```python
from build123d import *

# Parameters (mm, degrees)
BATON_DEPTH       = 2.54
SKETCH5_R         = 1.905
JOINER_HOLE_DEPTH = 2.54


with BuildPart() as part:
    # Sketch1 → baton (new body)
    with BuildSketch(Plane(origin=(0, 0, 0), x_dir=(1, 0, 0), z_dir=(0, 1, 0))):
        with BuildLine():
            Line((-12.7, 5.08), (12.7, 5.08))
            ThreePointArc((12.7, 5.08), (17.78, 0), (12.7, -5.08))
            Line((12.7, -5.08), (-12.7, -5.08))
            ThreePointArc((-12.7, -5.08), (-17.78, 0), (-12.7, 5.08))
        make_face()
    extrude(amount=BATON_DEPTH)

    # Sketch5 → joiner hole (cut)
    with BuildSketch(Plane(origin=(0, 2.54, 0), x_dir=(1, 0, 0), z_dir=(0, 1, 0))):
        with Locations(Location((13.97, 0, 0), (0, 0, 270))):
            Circle(SKETCH5_R)
    extrude(amount=-JOINER_HOLE_DEPTH, mode=Mode.SUBTRACT)


solid = part.part
```
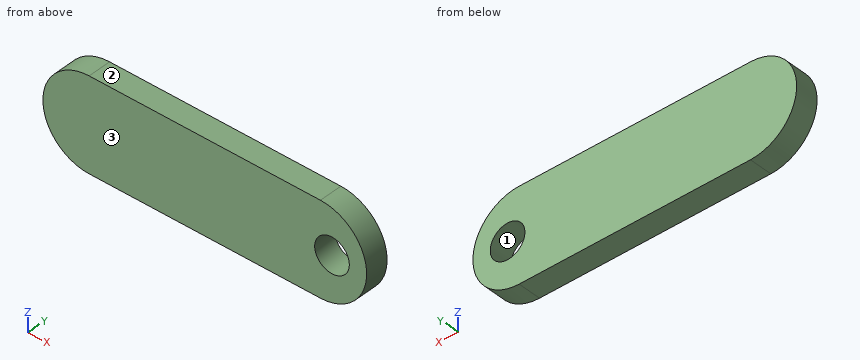
CAD build for the part. Positions are in the model's coordinates, mm. Face numbers are marked on the shaded views. Give positions to 0.01 mm unless a question says otherwise; leave off trailing zeros. Order: outer loops, then holes, each group sorted by start corner. A loop starts at its lowest first (then second) coordinate and runs counter-clockwise, first axis right, second up.
(1) Saw through at B-B, the plane y = 0.95. Give the cut face in (x, z) (3 decimals).
(2) Saw through at A-A, the plane z = 0. Give the cut face in (x, y) (3 decimals), then the cut area to 3 significant figures.
(3) Flat gauge pins, fed straight in: pin 1 (2.5 mm diameter, centred on x = 13.97, z = 0, fed in from -Y); pin 2 (1.5 mm diameter, centred on x = 2.5, z = 0, fed in from -Y). Where does each tip first touch, or does it go through?
(4) Saw through at D-D, the plane z = 2.5. Give the cut face in (x, y).
(5) Saw through at C-C, the plane x = 13.97. Give the cut face in (y, z) (3 decimals), then the cut area to 3 significant figures.
(6) Mould opens along Z. For the marked faces 1, 2 and 3 say: released by +Z, released by -Z, zero draft, split by the parting line, or undercut.
(7) Drill centre lines: L1, parallel to X at y = 1.95, z = 0 (3 decimals); L2, parallel to X at y = 1.35, z = 0.5; L3, parallel to X at y = 1, z = 4.5. Where is each one in solid material? Low to high.
Results found:
1. outline: (-12.7, -5.08) - (12.7, -5.08) arc R5.08 ccw to (12.7, 5.08) - (-12.7, 5.08) arc R5.08 ccw to start; hole circle Ø3.81 at (13.97, 0)
2. outline: (-17.78, 0) - (12.065, 0) - (12.065, 2.54) - (-17.78, 2.54) - close; (15.875, 0) - (17.78, 0) - (17.78, 2.54) - (15.875, 2.54) - close
2. area: 80.6 mm2
3. pin 1: passes through
3. pin 2: stops at y = 0
4. outline: (-17.12, 0) - (17.12, 0) - (17.12, 2.54) - (-17.12, 2.54) - close
5. outline: (0, -4.919) - (2.54, -4.919) - (2.54, -1.905) - (0, -1.905) - close; (0, 1.905) - (2.54, 1.905) - (2.54, 4.919) - (0, 4.919) - close
5. area: 15.3 mm2
6. face 1: undercut
6. face 2: released by +Z
6. face 3: zero draft
7. L1: x = -17.78 to 12.065, 15.875 to 17.78
7. L2: x = -17.76 to 12.13, 15.81 to 17.76
7. L3: x = -15.06 to 15.06
